Geometry: final body of the model. Coordinates: model frame, mm. A direction names the side the tool comes from. Give positions to 0.01 mm unless a question says otherwise; leave off trailing zeros. Write each loop counter-clockwise with the first axis right and the second up, starting at its lowest first coordinate (ties: lowest second). Pieces come first, ordered by that corner, then holes.
```python
from build123d import *

# Parameters (mm, degrees)
PAD_DEPTH       = 42
PAD001_DEPTH    = 18
SKETCH002_R     = 2
PAD002_DEPTH    = 3.5
SKETCH003_R     = 1.75
PAD003_DEPTH    = 6.5
SKETCH004_R     = 2
PAD004_DEPTH    = 9
FILLET_R        = 1
POCKET_DEPTH    = 5
SKETCH006_W     = 4.5
SKETCH006_H     = 12
POCKET001_DEPTH = 10
SKETCH007_W     = 1.5
SKETCH007_H     = 11
PAD005_DEPTH    = 9
CHAMFER_SIZE    = 0.2


with BuildPart() as part:
    # Sketch → Pad (new body)
    with BuildSketch(Plane.XY):
        with BuildLine():
            ThreePointArc((-14, 13.5), (-19.303301, 11.303301), (-21.5, 6))
            Line((-21.5, -6), (-21.5, 6))
            ThreePointArc((-21.5, -6), (-19.303301, -11.303301), (-14, -13.5))
            Line((14, -13.5), (-14, -13.5))
            ThreePointArc((14, -13.5), (19.303301, -11.303301), (21.5, -6))
            Line((21.5, 6), (21.5, -6))
            ThreePointArc((21.5, 6), (19.303301, 11.303301), (14, 13.5))
            Line((-14, 13.5), (14, 13.5))
        make_face()
    extrude(amount=PAD_DEPTH)

    # Sketch001 (on Face10 of Pad) → Pad001 (join)
    with BuildSketch(Plane.XY.offset(42)):
        with BuildLine():
            Line((-8.5, 6.5), (8.5, 6.5))
            ThreePointArc((13.107614, 4.593401), (10.993252, 6.004526), (8.5, 6.5))
            Line((13.107614, 4.593401), (17.353299, 0.353807))
            ThreePointArc((17.353299, -0.353807), (17.5, 0), (17.353299, 0.353807))
            Line((17.353299, -0.353807), (13.107614, -4.593401))
            ThreePointArc((8.5, -6.5), (10.993252, -6.004526), (13.107614, -4.593401))
            Line((8.5, -6.5), (-8.5, -6.5))
            ThreePointArc((-13.107614, -4.593401), (-10.993252, -6.004526), (-8.5, -6.5))
            Line((-17.353299, -0.353807), (-13.107614, -4.593401))
            ThreePointArc((-17.353299, 0.353807), (-17.5, 0), (-17.353299, -0.353807))
            Line((-17.353299, 0.353807), (-13.107614, 4.593401))
            ThreePointArc((-8.5, 6.5), (-10.993252, 6.004526), (-13.107614, 4.593401))
        make_face()
    extrude(amount=PAD001_DEPTH)

    # Sketch002 (on Face23 of Pad001) → Pad002 (join)
    with BuildSketch(Plane.XY.offset(60)):
        with Locations((-9.25, 0)):
            Circle(SKETCH002_R)
        with Locations((9.25, 0)):
            Circle(SKETCH002_R)
    extrude(amount=PAD002_DEPTH)

    # Sketch003 (on Face27 of Pad002) → Pad003 (join)
    with BuildSketch(Plane.XY.offset(63.5)):
        with Locations((9.25, 0)):
            Circle(SKETCH003_R)
        with Locations((-9.25, 0)):
            Circle(SKETCH003_R)
    extrude(amount=PAD003_DEPTH)

    # Sketch004 (on Face31 of Pad003) → Pad004 (join)
    with BuildSketch(Plane.XY.offset(70)):
        with Locations((9.25, 0)):
            Circle(SKETCH004_R)
        with Locations((-9.25, 0)):
            Circle(SKETCH004_R)
    extrude(amount=PAD004_DEPTH)

    # Fillet
    fillet_edges = [part.edges().sort_by_distance(p)[0] for p in [
        (-11.25, 0, 79),
        (7.25, 0, 79),
    ]]
    fillet(fillet_edges, radius=FILLET_R)

    # Sketch005 (on Face33 of Fillet) → Pocket (cut)
    with BuildSketch(Plane(origin=(0, 0, 0), x_dir=(1, 0, 0), z_dir=(0, 0, -1))):
        with BuildLine():
            ThreePointArc((-13.5, 12), (-18.096194, 10.096194), (-20, 5.5))
            Line((-20, -5.5), (-20, 5.5))
            ThreePointArc((-20, -5.5), (-18.096194, -10.096194), (-13.5, -12))
            Line((13.5, -12), (-13.5, -12))
            ThreePointArc((13.5, -12), (18.096194, -10.096194), (20, -5.5))
            Line((20, 5.5), (20, -5.5))
            ThreePointArc((20, 5.5), (18.096194, 10.096194), (13.5, 12))
            Line((-13.5, 12), (13.5, 12))
        make_face()
        with BuildLine():
            ThreePointArc((-13.5, 11.75), (-17.919417, 9.919417), (-19.75, 5.5))
            Line((-19.75, -5.5), (-19.75, 5.5))
            ThreePointArc((-19.75, -5.5), (-17.919417, -9.919417), (-13.5, -11.75))
            Line((13.5, -11.75), (-13.5, -11.75))
            ThreePointArc((13.5, -11.75), (17.919417, -9.919417), (19.75, -5.5))
            Line((19.75, 5.5), (19.75, -5.5))
            ThreePointArc((19.75, 5.5), (17.919417, 9.919417), (13.5, 11.75))
            Line((-13.5, 11.75), (13.5, 11.75))
        make_face(mode=Mode.SUBTRACT)
    extrude(amount=-POCKET_DEPTH, mode=Mode.SUBTRACT)

    # Sketch006 (on Face55 of Pocket) → Pocket001 (cut)
    with BuildSketch(Plane(origin=(0, 0, 0), x_dir=(1, 0, 0), z_dir=(0, 0, -1))):
        with Locations((-7.75, 0)):
            Rectangle(SKETCH006_W, SKETCH006_H)
    extrude(amount=-POCKET001_DEPTH, mode=Mode.SUBTRACT)

    # Sketch007 (on Face60 of Pocket001) → Pad005 (join)
    with BuildSketch(Plane(origin=(0, 0, 10), x_dir=(1, 0, 0), z_dir=(0, 0, -1))):
        with Locations((-6.75, 0)):
            Rectangle(SKETCH007_W, SKETCH007_H)
    extrude(amount=PAD005_DEPTH)

    # Chamfer
    chamfer_edges = [part.edges().sort_by_distance(p)[0] for p in [
        (-7.5, 0, 1),
        (-6.75, 5.5, 1),
        (-6, 0, 1),
        (-6.75, -5.5, 1),
    ]]
    chamfer(chamfer_edges, length=CHAMFER_SIZE)


solid = part.part
```
Item 1: Line query: L1, parallel to Z at x = 11, y = -11.5; L2, parallel to Z at x = -11, y = -0.5; L3, parallel to X at y = -1.75, z = 60.5. Output: solid intervals per line, ascending.
Found:
L1: z = 0 to 42
L2: z = 0 to 63.5, 70 to 78.57
L3: x = -10.22 to -8.28, 8.28 to 10.22
Item 2: Reachability of faces 1 (the face through (15.26, -2.444, 50.874)), 2 (the face through (11, 6, 51)), 3 (the face through (20, 0, 2)) from +Z, -Z, +X, -X, +Y, -Y: full face, straight path, thin tool, end or side. Return the list, or none.
Found:
face 1: +Z, +X, -Y
face 2: +Z, +X, +Y
face 3: -Z
Item 3: Section B-B, the plane z = 11. Return the cut outline in (x, y).
Found:
outline: (-21.5, -6) arc R7.5 ccw to (-14, -13.5) - (14, -13.5) arc R7.5 ccw to (21.5, -6) - (21.5, 6) arc R7.5 ccw to (14, 13.5) - (-14, 13.5) arc R7.5 ccw to (-21.5, 6) - close
Item 4: Section C-C, the plane y = 8. Return the cut outline in (x, z).
Found:
outline: (-21.23, 0) - (-19.5, 0) - (-19.5, 5) - (-19.23, 5) - (-19.23, 0) - (19.23, 0) - (19.23, 5) - (19.5, 5) - (19.5, 0) - (21.23, 0) - (21.23, 42) - (-21.23, 42) - close
Item 5: Section A-A, the plane x = 1. Return the cut outline in (y, z).
Found:
outline: (-13.5, 0) - (-12, 0) - (-12, 5) - (-11.75, 5) - (-11.75, 0) - (11.75, 0) - (11.75, 5) - (12, 5) - (12, 0) - (13.5, 0) - (13.5, 42) - (6.5, 42) - (6.5, 60) - (-6.5, 60) - (-6.5, 42) - (-13.5, 42) - close
Item 6: Section D-D, the plane z = 54. Return the cut outline in (x, y).
Found:
outline: (-17.35, -0.35) - (-13.11, -4.59) arc R6.52 ccw to (-8.5, -6.5) - (8.5, -6.5) arc R6.52 ccw to (13.11, -4.59) - (17.35, -0.35) arc R0.5 ccw to (17.35, 0.35) - (13.11, 4.59) arc R6.52 ccw to (8.5, 6.5) - (-8.5, 6.5) arc R6.52 ccw to (-13.11, 4.59) - (-17.35, 0.35) arc R0.5 ccw to start
Item 7: Pull-direction query (Z, two-part tool) for faces 4 (the face through (-7.5, 0, 6)), 5 (the face through (-7.581, 0.526, 66.704)); classes: +Z half, -Z half, draft (parallel to the pull), parting line (faces both ways), or undercut.
Found:
face 4: draft
face 5: undercut
Item 8: Pin query (flat end, axial travel): pin 1 Ø0.5 at (x, y) = (-6.5, -1) entering from -Z; pin 2 Ø8.5 at (x, z) = (-3, 48) entering from +Y; pin 3 Ø8.5 at (x, z) = (2.5, 54.5) entering from -Y. Return the tip coordinate at first contact, or that it passes through.
Found:
pin 1: stops at z = 1
pin 2: stops at y = 6.5
pin 3: stops at y = -6.5
